```python
from build123d import *

# Parameters (mm, degrees)
SKETCH1_W           = 240
SKETCH1_H           = 160
BOSS_EXTRUDE1_DEPTH = 2
SKETCH5_R           = 1.5
CUT_EXTRUDE2_DEPTH  = 4
SKETCH6_W           = 240
SKETCH6_H           = 160
SKETCH6_W_2         = 237
SKETCH6_H_2         = 157
BOSS_EXTRUDE2_DEPTH = 40
SKETCH7_W           = 7
SKETCH7_H           = 7
BOSS_EXTRUDE3_DEPTH = 40
SKETCH8_R           = 2.9
CUT_EXTRUDE3_DEPTH  = 6.2


with BuildPart() as part:
    # Sketch1 → Boss-Extrude1 (new body)
    with BuildSketch(Plane.XY):
        Rectangle(SKETCH1_W, SKETCH1_H)
    extrude(amount=BOSS_EXTRUDE1_DEPTH)

    # Sketch5 → Cut-Extrude2 (cut)
    with BuildSketch(Plane.XY.offset(2)):
        with Locations((-110, 70)):
            Circle(SKETCH5_R)
        with Locations((0, 70)):
            Circle(SKETCH5_R)
        with Locations((110, 70)):
            Circle(SKETCH5_R)
        Circle(SKETCH5_R)
        with Locations((110, 0)):
            Circle(SKETCH5_R)
        with Locations((0, -70)):
            Circle(SKETCH5_R)
        with Locations((110, -70)):
            Circle(SKETCH5_R)
        with Locations((-110, 0)):
            Circle(SKETCH5_R)
        with Locations((-110, -70)):
            Circle(SKETCH5_R)
    extrude(amount=-CUT_EXTRUDE2_DEPTH, mode=Mode.SUBTRACT)

    # Sketch6 → Boss-Extrude2 (add)
    with BuildSketch(Plane(origin=(0, 0, 0), x_dir=(-1, 0, 0), z_dir=(0, 0, -1))):
        Rectangle(SKETCH6_W, SKETCH6_H)
        Rectangle(SKETCH6_W_2, SKETCH6_H_2, mode=Mode.SUBTRACT)
    extrude(amount=BOSS_EXTRUDE2_DEPTH)

    # Sketch7 → Boss-Extrude3 (add)
    with BuildSketch(Plane(origin=(0, 0, 0), x_dir=(-1, 0, 0), z_dir=(0, 0, -1))):
        with Locations((115, -75)):
            Rectangle(SKETCH7_W, SKETCH7_H)
        with Locations((115, 75)):
            Rectangle(SKETCH7_W, SKETCH7_H)
        with Locations((-115, 75)):
            Rectangle(SKETCH7_W, SKETCH7_H)
        with Locations((-115, -75)):
            Rectangle(SKETCH7_W, SKETCH7_H)
    extrude(amount=BOSS_EXTRUDE3_DEPTH)

    # Sketch8 → Cut-Extrude3 (cut)
    with BuildSketch(Plane(origin=(0, 0, -40), x_dir=(-1, 0, 0), z_dir=(0, 0, -1))):
        with Locations((116, -76)):
            Circle(SKETCH8_R)
        with Locations((116, 76)):
            Circle(SKETCH8_R)
        with Locations((-116, 76)):
            Circle(SKETCH8_R)
        with Locations((-116, -76)):
            Circle(SKETCH8_R)
    extrude(amount=-CUT_EXTRUDE3_DEPTH, mode=Mode.SUBTRACT)


solid = part.part
```
Could you check a few things on this model? Use its own coordinates, in mm. A direction names the side the tool comes from. Round coordinates to 2 decimals unless told otherwise and drop trailing zeros. Loops run counter-clockwise (first coordinate to the right, second up) from the corner with the lowest first, then second, coordinate; pieces in that order, holes last. Notation, with made-up numbers: (75.5, 22.5) -> (128.5, 22.5) arc R20 cw to (128.5, 35.5) -> close; hole circle Ø7 at (-19.5, -6.75). An arc over 180 degrees is marked (long way). One line per question, with ' | ' between items.
(1) For pin 1 Ø1.7 at (x, y) = (117, -75) entering from -Z; pin 2 Ø6.5 at (x, y) = (-116, -76) entering from -Z; pin 3 Ø3 at (x, y) = (53.5, -19) entering from -Z, each with a flat end and sliding along its axis, tell me the tip position at first contact or that it passes through.
Model answer:
pin 1: stops at z = -33.8 | pin 2: stops at z = -40 | pin 3: stops at z = 0
(2) Thinking about a two-plate mould opening in X: for faces 3 (the face through (-2, 1, 0)), 4 (the face through (2, -80, -19)), 5 (the face through (-120, -1, -19)), which applies, released by +X, released by -X, zero draft, split by the parting line, or undercut?
Model answer:
face 3: undercut | face 4: zero draft | face 5: released by -X
(3) If we section it at B-B on x = -51: List the corners of the cut face in (y, z) for me, and give its area (3 significant figures).
Model answer:
outline: (-80, -40) -> (-78.5, -40) -> (-78.5, 0) -> (78.5, 0) -> (78.5, -40) -> (80, -40) -> (80, 2) -> (-80, 2) -> close | area: 440 mm^2
(4) For faces 1 (the face through (-111.5, 75, -20)), 2 (the face through (-2, 1, 2)), which set-ups out of +Z, -Z, +X, -X, +Y, -Y let a thin tool reach every point of the face, with its end or its side?
Model answer:
face 1: -Z | face 2: +Z, +X, -X, +Y, -Y
(5) If we section it at A-A on z = -20.5: List the corners of the cut face in (x, y) for me, and give its area (3 significant figures).
Model answer:
outline: (-120, -80) -> (120, -80) -> (120, 80) -> (-120, 80) -> close; hole (-118.5, -71.5) -> (-111.5, -71.5) -> (-111.5, -78.5) -> (111.5, -78.5) -> (111.5, -71.5) -> (118.5, -71.5) -> (118.5, 71.5) -> (111.5, 71.5) -> (111.5, 78.5) -> (-111.5, 78.5) -> (-111.5, 71.5) -> (-118.5, 71.5) -> close | area: 1,390 mm^2
(6) If I drill on probe 1 along Y at (x, z) = (-110, 1.5); probe 2 along X at (y, z) = (-70, 1); probe 3 along Y at (x, z) = (-64.5, -22.5), over which ranges is the centre line in solid material (lowest first)?
Model answer:
probe 1: y = -80 to -71.5, -68.5 to -1.5, 1.5 to 68.5, 71.5 to 80 | probe 2: x = -120 to -111.5, -108.5 to -1.5, 1.5 to 108.5, 111.5 to 120 | probe 3: y = -80 to -78.5, 78.5 to 80
(7) If we section it at D-D on y = -40.5: List the corners of the cut face in (x, z) for me, and give its area (3 significant figures).
Model answer:
outline: (-120, -40) -> (-118.5, -40) -> (-118.5, 0) -> (118.5, 0) -> (118.5, -40) -> (120, -40) -> (120, 2) -> (-120, 2) -> close | area: 600 mm^2
(8) If we section it at C-C on y = -76: List the corners of the cut face in (x, z) for me.
Model answer:
outline: (-120, -40) -> (-118.9, -40) -> (-118.9, -33.8) -> (-113.1, -33.8) -> (-113.1, -40) -> (-111.5, -40) -> (-111.5, 0) -> (111.5, 0) -> (111.5, -40) -> (113.1, -40) -> (113.1, -33.8) -> (118.9, -33.8) -> (118.9, -40) -> (120, -40) -> (120, 2) -> (-120, 2) -> close
